from build123d import *

# Parameters (mm, degrees)
F0_R     = 0.75
F1_DEPTH = 3


with BuildPart() as f1:
    # F0 (on Front) → F1 (new body)
    with BuildSketch(Plane.XZ):
        with BuildLine():
            ThreePointArc((3.076821, -1.25), (3.960705, -0.883883), (4.326821, 0))
            ThreePointArc((4.326821, 0), (3.960705, 0.883883), (3.076821, 1.25))
            ThreePointArc((3.076821, 1.25), (1.826821, 0), (3.076821, -1.25))
        make_face()
        with Locations((3.076821, 0)):
            Circle(F0_R, mode=Mode.SUBTRACT)
        with BuildLine():
            ThreePointArc((3.076821, -1.25), (1.826821, 0), (3.076821, 1.25))
            Line((3.076821, 1.25), (-1.902765, 1.25))
            ThreePointArc((-1.902765, 1.25), (-2.529328, 1.547448), (-2.694943, 2.220968))
            Line((-2.694943, 2.220968), (-3.694943, 2.220968))
            ThreePointArc((-3.694943, 2.220968), (-4.038078, 2.084641), (-4.194099, 1.75))
            Line((-4.194099, 1.75), (-4.194099, 1.691935))
            Line((-4.194099, 1.691935), (-4.194099, 1.25))
            ThreePointArc((-4.194099, 1.25), (-2.944099, 0), (-4.194099, -1.25))
            Line((-4.194099, -1.25), (-4.194099, -1.691935))
            Line((-4.194099, -1.691935), (-4.194099, -1.75))
            ThreePointArc((-4.194099, -1.75), (-4.038078, -2.084641), (-3.694943, -2.220968))
            Line((-3.694943, -2.220968), (-2.694943, -2.220968))
            ThreePointArc((-2.694943, -2.220968), (-2.529328, -1.547448), (-1.902765, -1.25))
            Line((-1.902765, -1.25), (3.076821, -1.25))
        make_face()
        with BuildLine():
            ThreePointArc((-1.694099, 0.5), (-1.688425, 0.499968), (-1.682752, 0.499871))
            Line((-1.682752, 0.499871), (0.811253, 0.471568))
            ThreePointArc((0.811253, 0.471568), (1.277499, 0), (0.811253, -0.471568))
            Line((0.811253, -0.471568), (-1.682752, -0.499871))
            ThreePointArc((-1.682752, -0.499871), (-1.688425, -0.499968), (-1.694099, -0.5))
            ThreePointArc((-1.694099, -0.5), (-2.194099, 0), (-1.694099, 0.5))
        make_face(mode=Mode.SUBTRACT)
        with BuildLine():
            Line((-4.194099, 1.691935), (-4.194099, 1.75))
            ThreePointArc((-4.194099, 1.75), (-4.194943, 1.720968), (-4.194099, 1.691935))
        make_face()
        with BuildLine():
            ThreePointArc((-4.194099, -1.691935), (-4.194943, -1.720968), (-4.194099, -1.75))
            Line((-4.194099, -1.75), (-4.194099, -1.691935))
        make_face()
    extrude(amount=F1_DEPTH)


solid = f1.part
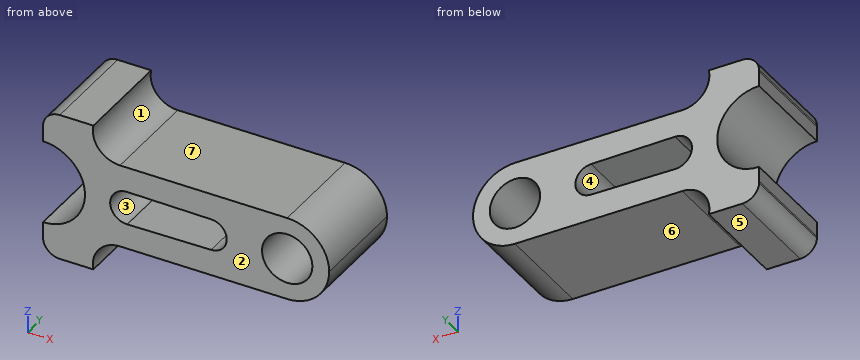
Model file for the job. Use its own axes, mm. Face numbers are marked on the shaded views. A direction names the side the tool comes from. Coordinates: 2 decimals unless noted, no trailing zeros. Loops run counter-clockwise (first coordinate to the right, second up) from the corner with the lowest first, then second, coordinate; pieces in that order, holes last. Notation, with made-up numbers: (64, -24) -> (113, -24) arc R24 cw to (113, 12) -> close; hole circle Ø6 at (20, 87). An arc over 180 degrees is marked (long way). Use one line per item in the form item = value. Start each with the question number.
(1) Cut at B-B on x = -3.5. Give the cut face in (y, z), and give its area (3 significant figures).
(2) Cut at D-D on x = 1.75. Give the cut face in (y, z).
(3) Tool access for the marked faces 5, 6 and 7: list every direction of +Z, -Z, +X, -X, +Y, -Y with a clear straight run to the whole face (end or side of a thin tool).
(4) Cut at C-C on z = 0.65. Give the cut face in (x, y), and give its area (3 significant figures).
(5) Probe probe 1 along X at (y, z) = (-1.85, -0.05); probe 2 along X at (y, z) = (-1.55, 0.3); probe 3 along Z at (x, y) = (-1, -1.25). List the from-to ranges inside material, lowest first. Write a range as from..to.
(6) Pull direction X, two halves, no side cores. Call the marked faces 1, 2, 3 and 4: pulls with the +X half, pulls with the -X half, needs draft (parallel to the pull), parting line crosses it, or undercut.
(7) Cut at A-A on y = -0.6. Give the number of separate pieces and of enclosed holes in the cut face, and give its area (3 significant figures).
Values:
q1.outline = (-3, -2.22) -> (0, -2.22) -> (0, -1.04) -> (-3, -1.04) -> close; (-3, 1.04) -> (0, 1.04) -> (0, 2.22) -> (-3, 2.22) -> close
q1.area = 7.09 mm2
q2.outline = (-3, -1.25) -> (0, -1.25) -> (0, 1.25) -> (-3, 1.25) -> close
q3.face_5 = -Z, +X, -X, +Y, -Y
q3.face_6 = -Z, +X, +Y, -Y
q3.face_7 = +Z, +X, +Y, -Y
q4.outline = (-3.13, -3) -> (2.7, -3) -> (2.7, 0) -> (-3.13, 0) -> close; (3.45, -3) -> (4.14, -3) -> (4.14, 0) -> (3.45, 0) -> close
q4.area = 19.6 mm2
q5.probe_1 = -2.95..-2.19, 1.27..2.33, 3.83..4.33
q5.probe_2 = -2.98..-2.09, 1.17..2.39, 3.76..4.29
q5.probe_3 = -1.25..-0.49, 0.49..1.25
q6.face_1 = pulls with the +X half
q6.face_2 = needs draft
q6.face_3 = undercut
q6.face_4 = undercut
q7.separate_pieces = 1
q7.enclosed_holes = 2
q7.area = 16.3 mm2
